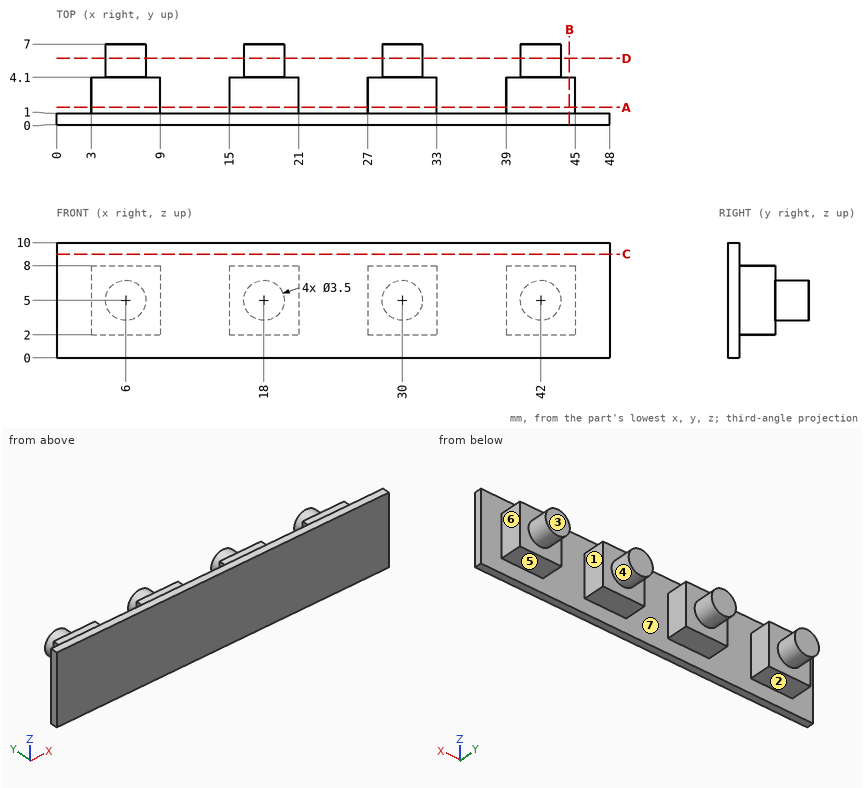
Check sheet for the drawn part. Datum: minimum x, y, z corner. Units: mm. A direction names the side the tool comes from. Round coordinates to 2 decimals unless told otherwise and drop trailing zeros. Order: outer loops, then holes, each group sorted by start corner. A loop starts at its lowest first (then second) coordinate and runs counter-clockwise, first axis right, second up. Notation, with made-up numbers: (86.5, -30.5) -> (129.5, -30.5) arc R13 cw to (129.5, -12.5) -> close; hole circle Ø4 at (45, 27). An arc over 180 degrees is marked (long way). Put each result on its own line as item: value. Start each with the question number.
(1) Section check D-D (y = 5.75). Enter the section's corners in (x, z).
(2) Section check A-A (y = 1.5). Enter the section's corners in (x, z).
(3) Depth check by flat-ended pin: pin 1 Ø2.5 at (x, y) = (18.5, 3) entering from -Z; pin 2 Ø4 at (x, y) = (8, 4) entering from +Z; pin 3 Ø1.5 at (y, z) = (2.5, 4) entering from +X. Enter the tip coordinate at first touch or a pass-through.
(4) Draft check along X on the marked faces 5, 6 and 7. Enter one of: +X half, -X half, draft (parallel to the pull), parting line (faces both ways), or undercut.
(5) Section check C-C (z = 9). Enter the section's corners in (x, y), then the cut area to 3 significant figures.
(6) Material ranges on line 1 along X through (y, z) = (2.5, 4.25); line 2 along X through (y, z) = (4.75, 5); line 3 along Y through (x, z) = (43, 8.25), recorded low to high.
(7) Section check B-B (x = 44.5). Enter the section's corners in (y, z), then the cut area to 3 significant figures.
(8) Tool access check on the marked faces 1, 2, 3 and 4. Record the directions out of +Z, -Z, +X, -X, +Y, -Y that give a thin tool (end or side, any length) a straight path to the whole face; none if there is none.
Completed:
1. outline: circle Ø3.5 at (6, 5); circle Ø3.5 at (18, 5); circle Ø3.5 at (30, 5); circle Ø3.5 at (42, 5)
2. outline: (3, 2) -> (9, 2) -> (9, 8) -> (3, 8) -> close; (15, 2) -> (21, 2) -> (21, 8) -> (15, 8) -> close; (27, 2) -> (33, 2) -> (33, 8) -> (27, 8) -> close; (39, 2) -> (45, 2) -> (45, 8) -> (39, 8) -> close
3. pin 1: stops at z = 2
3. pin 2: stops at z = 8
3. pin 3: stops at x = 45
4. face 5: draft
4. face 6: +X half
4. face 7: undercut
5. outline: (0, 0) -> (48, 0) -> (48, 1) -> (0, 1) -> close
5. area: 48.0 mm2
6. line 1: x = 3 to 9, 15 to 21, 27 to 33, 39 to 45
6. line 2: x = 4.25 to 7.75, 16.25 to 19.75, 28.25 to 31.75, 40.25 to 43.75
6. line 3: y = 0 to 1
7. outline: (0, 0) -> (1, 0) -> (1, 2) -> (4.1, 2) -> (4.1, 8) -> (1, 8) -> (1, 10) -> (0, 10) -> close
7. area: 28.6 mm2
8. face 1: +Z, -Z, +Y
8. face 2: -Z, +X, -X, +Y
8. face 3: +Z, -Z, +X, -X, +Y
8. face 4: +Y
